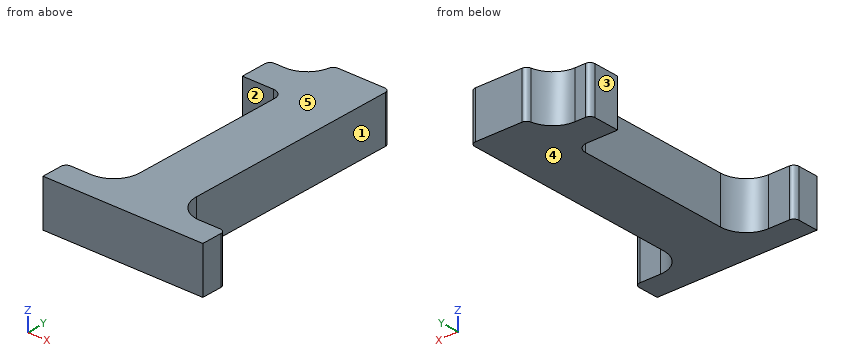
from build123d import *

# Parameters (mm, degrees)
F1_DEPTH = 4.5
F2_R     = 1


with BuildPart() as f1:
    # F0 (on Top) → F1 (new body, symmetric)
    with BuildSketch(Plane.XY):
        with BuildLine():
            Line((-5.5, -26.5), (5.5, -26.5))
            Line((5.5, -26.5), (15.5, -26.5))
            Line((15.5, -26.5), (15.5, -22.5))
            ThreePointArc((15.5, -22.5), (15.2071067812, -21.7928932188), (14.5, -21.5))
            Line((14.5, -21.5), (10.5, -21.5))
            ThreePointArc((10.5, -21.5), (6.9644660941, -20.0355339059), (5.5, -16.5))
            Line((5.5, -16.5), (5.5, 26.5))
            Line((5.5, 26.5), (-5.5, 26.5))
            ThreePointArc((-5.5, 26.5), (-6.9644660941, 22.9644660941), (-10.5, 21.5))
            Line((-10.5, 21.5), (-12.5, 21.5))
            ThreePointArc((-12.5, 21.5), (-13.2071067812, 21.2071067812), (-13.5, 20.5))
            Line((-13.5, 20.5), (-13.5, 15.5))
            Line((-13.5, 15.5), (-7.5, 15.5))
            ThreePointArc((-7.5, 15.5), (-6.0857864376, 14.9142135624), (-5.5, 13.5))
            Line((-5.5, 13.5), (-5.5, -16.5))
            ThreePointArc((-5.5, -16.5), (-6.9644660941, -20.0355339059), (-10.5, -21.5))
            Line((-10.5, -21.5), (-14.5, -21.5))
            ThreePointArc((-14.5, -21.5), (-15.2071067812, -21.7928932188), (-15.5, -22.5))
            Line((-15.5, -22.5), (-15.5, -26.5))
            Line((-15.5, -26.5), (-5.5, -26.5))
        make_face()
    extrude(amount=F1_DEPTH, both=True)

    # F2
    f2_edges = [f1.edges().sort_by_distance(p)[0] for p in [
        (5.5, 26.5, 0),
        (-5.5, 26.5, 0),
    ]]
    fillet(f2_edges, radius=F2_R)


solid = f1.part
The model under review builds one solid part; all positions refer to its coordinate system, in mm. Face numbers are marked on the shaded views. A direction names the side the tool comes from. Coordinates: 2 decimals unless noted, no trailing zeros. Order: outer loops, then holes, each group sorted by start corner. A loop starts at its lowest first (then second) coordinate and runs counter-clockwise, first axis right, second up. Notation, with made-up numbers: (-3.5, 42) -> (46.5, 42) arc R19 cw to (46.5, 74) -> close; hole circle Ø1 at (52.25, 81.5). An arc over 180 degrees is marked (long way). Answer in a Markdown table with one row per item.
(1) Machinability: for the marked faces 1, 2, 3, 4 and 5, which of the approach directions +Z, -Z, +X, -X, +Y, -Y give a long, thin tool a straight path to every point of the face, cutting with its end or side? Answer none if there is none.
Answers:
| item | result |
|---|---|
| face 1 | +Z, -Z, +X, +Y |
| face 2 | +Z, -Z, -X |
| face 3 | +Z, -Z, -X, +Y |
| face 4 | -Z, +X, -X, +Y, -Y |
| face 5 | +Z, +X, -X, +Y, -Y |
(2) Consider section D-D (x = 13.5). Write out the cut boundary in (y, z), plus the area to 3 significant figures.
Answers:
| item | result |
|---|---|
| outline | (-26.5, -4.5) -> (-21.5, -4.5) -> (-21.5, 4.5) -> (-26.5, 4.5) -> close |
| area | 45.0 mm² |
(3) Consider section B-B (z = 4). Write out the cut boundary in (x, y), plus the area to 3 significant figures.
Answers:
| item | result |
|---|---|
| outline | (-15.5, -26.5) -> (15.5, -26.5) -> (15.5, -22.5) arc R1 ccw to (14.5, -21.5) -> (10.5, -21.5) arc R5 cw to (5.5, -16.5) -> (5.5, 25.5) arc R1 ccw to (4.5, 26.5) -> (-4.58, 26.5) arc R1 ccw to (-5.57, 25.67) arc R5 cw to (-10.5, 21.5) -> (-12.5, 21.5) arc R1 ccw to (-13.5, 20.5) -> (-13.5, 15.5) -> (-7.5, 15.5) arc R2 cw to (-5.5, 13.5) -> (-5.5, -16.5) arc R5 cw to (-10.5, -21.5) -> (-14.5, -21.5) arc R1 ccw to (-15.5, -22.5) -> close |
| area | 747 mm² |
(4) Consider section C-C (y = 16.5). Write out the cut boundary in (x, z), plus the area to 3 significant figures.
Answers:
| item | result |
|---|---|
| outline | (-13.5, -4.5) -> (5.5, -4.5) -> (5.5, 4.5) -> (-13.5, 4.5) -> close |
| area | 171 mm² |
(5) Insertion check: pin 1 (5 mm diameter, centred on y = 8.5, z = 0.5, fed in from +X); pin 2 (5 mm diameter, centred on y = 3.5, z = -1, fed in from -X); pin 3 (1.2 mm diameter, centred on x = 12, z = -1.5, fed in from +Y). Each pin has a flat end and moves straight along its axis. Give the tip position at first contact, or say it passes through.
Answers:
| item | result |
|---|---|
| pin 1 | x = 5.5 |
| pin 2 | x = -5.5 |
| pin 3 | y = -21.5 |
(6) Wall thickness on line 1 along Y through (x, z) = (-11, -0.25); line 2 along X through (y, z) = (-15, -1.5); line 3 along Y through (x, z) = (14.5, 2.5): over which ranges is each line inside the solid? List them lowest first.
Answers:
| item | result |
|---|---|
| line 1 | -26.5 to -21.5, 15.5 to 21.5 |
| line 2 | -5.5 to 5.5 |
| line 3 | -26.5 to -21.5 |
(7) Consider section A-A (x = -13). Write out the cut boundary in (y, z).
Answers:
| item | result |
|---|---|
| outline | (-26.5, -4.5) -> (-21.5, -4.5) -> (-21.5, 4.5) -> (-26.5, 4.5) -> close; (15.5, -4.5) -> (21.37, -4.5) -> (21.37, 4.5) -> (15.5, 4.5) -> close |
